from build123d import *

# Parameters (mm, degrees)
F0_W     = 11
F0_H     = 11
F2_W     = 9
F2_H     = 9
F6_ANGLE = 45


with BuildPart() as f3:
    # F0 (on Top) → F3 section 0
    with BuildSketch(Plane.XY):
        Rectangle(F0_W, F0_H)
    # F2 (on offset) → F3 section 1
    with BuildSketch(Plane.XY.offset(-4)):
        Rectangle(F2_W, F2_H)
    loft()

    # F4 (on Front) → F5 (revolve, cut)
    with BuildSketch(Plane.XZ):
        with BuildLine():
            Line((0, -4), (2.2, -4))
            Line((2.2, -4), (2.2, -2))
            ThreePointArc((2.2, -2), (2.414105, -1.193774), (3, -0.6))
            Line((3, -0.6), (3, 0))
            Line((3, 0), (0, 0))
            Line((0, 0), (0, -4))
        make_face()
    revolve(axis=Axis((0, 0, -1.994932), (0, 0, -1)), mode=Mode.SUBTRACT)


with BuildPart() as f3_1:
    # F6: moved
    add(f3.part.rotate(Axis((0, 0, -2), (0, 0, -1)), F6_ANGLE))


solid = f3_1.part
Could you check a few things on this model? Use its own coordinates, in mm. Round coordinates to 2 decimals unless told otherwise and drop trailing zeros. Write item = value, one per line.
1) I need wall thicknesses on line 1 along X through (y, z) = (-2.25, -1.1); line 2 along X through (y, z) = (-1, -0.5); line 3 along X through (y, z) = (6.25, -3.7). Which ranges of each line are inside material? Lowest first, please. Write a range as from..to.
Computed:
line_1 = -5.14..-1.02, 1.02..5.14
line_2 = -6.6..-2.83, 2.83..6.6
line_3 = -0.22..0.22
2) If we mould it in two halves opening along Y, with no side actions, what happens to faces 1 (the flat face through (-0.1, -3.3, 0)), 2 (the cylindrical face through (1.61, 2.53, -0.3)), 3 (the cylindrical face through (1.02, -1.95, -2.99))? For each: pulls with the +Y half, pulls with the -Y half, needs draft (parallel to the pull), parting line crosses it, or undercut.
Computed:
face_1 = needs draft
face_2 = undercut
face_3 = undercut
3) I'm going to push flat-ended pins straight in: P1, Ø1, axis at x = 5, z = -0.5, coming from the -Y side; P2, Ø1.5, axis at y = 5, z = -2.5, coming from the +X side; P3, Ø1, axis at x = 5, z = -1, coming from the -Y side. Where does each tip first touch, or does it pass through?
Computed:
P1 = -3.13
P2 = 2.69
P3 = -2.95
